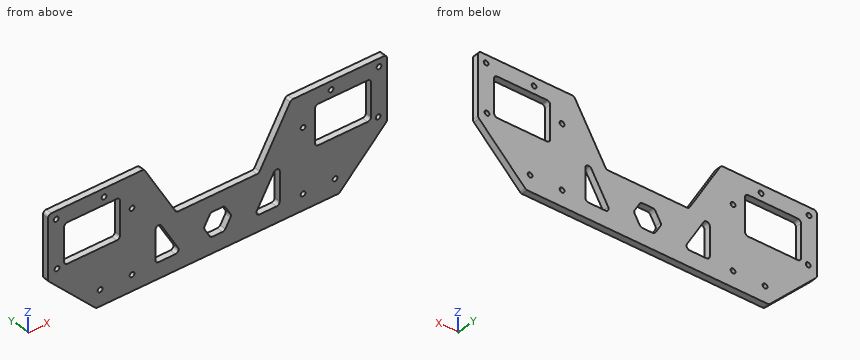
```python
from build123d import *

# Parameters (mm, degrees)
EXTRUDE_1_DEPTH     = 4
SKETCH_2_W          = 35
SKETCH_2_H          = 25
CUT_EXTRUDE_1_DEPTH = 4
SKETCH_3_R          = 1.5
CUT_EXTRUDE_2_DEPTH = 4
CUT_EXTRUDE_3_DEPTH = 4
FILLET_1_R          = 2


with BuildPart() as part:
    # 草图1 → 凸台-拉伸1 (new body)
    with BuildSketch(Plane(origin=(0, 0, 0), x_dir=(1, 0, 0), z_dir=(0, 1, 0))):
        Polygon((0, 0), (51.585481157, 0), (71.792740578, -35), (131.792740578, -35), (131.792740578, 5), (101.792740578, 35), (-50.207259422, 35), (-80.207259422, 5), (-80.207259422, -35), (-20.207259422, -35), align=None)
    extrude(amount=EXTRUDE_1_DEPTH)

    # 草图2 → 切除-拉伸1 (cut)
    with BuildSketch(Plane(origin=(0, 4, 0), x_dir=(1, 0, 0), z_dir=(0, 1, 0))):
        with Locations((-52.707259422, -12.5)):
            Rectangle(SKETCH_2_W, SKETCH_2_H)
        with Locations((104.292740578, -12.5)):
            Rectangle(SKETCH_2_W, SKETCH_2_H)
    extrude(amount=-CUT_EXTRUDE_1_DEPTH, mode=Mode.SUBTRACT)

    # 草图3 → 切除-拉伸2 (cut)
    with BuildSketch(Plane(origin=(0, 4, 0), x_dir=(1, 0, 0), z_dir=(0, 1, 0))):
        with Locations(Location((-75.207259422, -30, 0), (0, 0, 270))):
            Circle(SKETCH_3_R)
        with Locations(Location((-45.207259422, -29.79681333, 0), (0, 0, 270))):
            Circle(SKETCH_3_R)
        with Locations(Location((-74.668557439, 0, 0), (0, 0, 270))):
            Circle(SKETCH_3_R)
        with Locations(Location((126.254038596, 0, 0), (0, 0, 90))):
            Circle(SKETCH_3_R)
        with Locations(Location((96.792740578, -29.79681333, 0), (0, 0, 90))):
            Circle(SKETCH_3_R)
        with Locations(Location((126.792740578, -30, 0), (0, 0, 90))):
            Circle(SKETCH_3_R)
        with Locations(Location((-27.707259422, -15, 0), (0, 0, 270))):
            Circle(SKETCH_3_R)
        with Locations(Location((-47.707259422, 25, 0), (0, 0, 270))):
            Circle(SKETCH_3_R)
        with Locations(Location((-27.707259422, 25, 0), (0, 0, 270))):
            Circle(SKETCH_3_R)
        with Locations(Location((79.292740578, -15, 0), (0, 0, 90))):
            Circle(SKETCH_3_R)
        with Locations(Location((99.292740578, 25, 0), (0, 0, 90))):
            Circle(SKETCH_3_R)
        with Locations(Location((79.292740578, 25, 0), (0, 0, 90))):
            Circle(SKETCH_3_R)
    extrude(amount=-CUT_EXTRUDE_2_DEPTH, mode=Mode.SUBTRACT)

    # 草图4 → 切除-拉伸3 (cut)
    with BuildSketch(Plane(origin=(0, 4, 0), x_dir=(1, 0, 0), z_dir=(0, 1, 0))):
        Polygon((34.452994616, 17.5), (30.122867597, 25), (21.462613559, 25), (17.132486541, 17.5), (21.462613559, 10), (30.122867597, 10), align=None)
        Polygon((48.698729811, 25), (64.698729811, 25), (64.698729811, -2.712812921), align=None)
        Polygon((-13.113248654, 25), (-13.113248654, -2.712812921), (2.886751346, 25), align=None)
    extrude(amount=-CUT_EXTRUDE_3_DEPTH, mode=Mode.SUBTRACT)

    # 圆角1
    fillet_1_edges = [part.edges().sort_by_distance(p)[0] for p in [
        (34.452994616, 2, -17.5),
        (30.122867597, 2, -10),
        (21.462613559, 2, -10),
        (17.132486541, 2, -17.5),
        (21.462613559, 2, -25),
        (30.122867597, 2, -25),
        (64.698729811, 2, -25),
        (64.698729811, 2, 2.712812921),
        (48.698729811, 2, -25),
        (-13.113248654, 2, -25),
        (2.886751346, 2, -25),
        (-13.113248654, 2, 2.712812921),
        (-20.207259422, 2, 35),
        (-80.207259422, 2, 35),
        (-80.207259422, 2, -5),
        (-50.207259422, 2, -35),
        (101.792740578, 2, -35),
        (131.792740578, 2, -5),
        (131.792740578, 2, 35),
        (71.792740578, 2, 35),
        (51.585481157, 2, 0),
        (0, 2, 0),
        (-70.207259422, 2, 25),
        (-70.207259422, 2, 0),
        (-35.207259422, 2, 0),
        (-35.207259422, 2, 25),
        (121.792740578, 2, 0),
        (121.792740578, 2, 25),
        (86.792740578, 2, 25),
        (86.792740578, 2, 0),
    ]]
    fillet(fillet_1_edges, radius=FILLET_1_R)


solid = part.part
```
Design review of the part built by this model. Coordinates are the model's own, in mm. Give positions to 0.01 mm unless a question says otherwise; leave off trailing zeros. Return JSON: item names as keys, results as strings. Group by question number.
(1) To check wall thickness, follow probe 1 along X at (y, z) = (2.25, 24.5); probe 2 along X at (y, z) = (0.9, -6); probe 3 along X at (y, z) = (2.8, 30). State the ranges of each line that lie inside material, in increasing order.
(2) Insertion check: pin 1 (2.5 mm diameter, centred on x = 79.29, z = 15, fed in from +Y); pin 2 (1.2 mm diameter, centred on x = 112, y = 1, fed in from -Z). Each pin has a flat end and moves straight along its axis. Give the tip position at first contact, or say it passes through.
(3) We need section A-A, the plane y = 1.85. Give the number of separate pieces and of enclosed holes in the cut face, then the cut area to 3 significant figures.
Reported:
{
 "1": {"probe 1": "x = -80.21 to -69.53, -35.88 to -14.15, 65.73 to 87.47, 121.12 to 131.79", "probe 2": "x = -79.21 to -13.11, -8.08 to 59.67, 64.7 to 130.79", "probe 3": "x = -80.21 to -76.71, -73.71 to -46.69, -43.72 to -17.32, 68.91 to 95.31, 98.28 to 125.29, 128.29 to 131.79"},
 "2": {"pin 1": "passes through", "pin 2": "stops at z = -25.39"},
 "3": {"separate pieces": "1", "enclosed holes": "17", "area": "8,990 mm2"}
}
